Source: CAD feature listing. Evaluate the final solid. Frame: model axes, mm. Round coordinates to 2 decimals unless told otherwise and drop trailing zeros. Write each loop counter-clockwise with the first axis right and the second up, starting at its lowest first coordinate (ties: lowest second). Pieces come first, ordered by that corner, then holes. Notation, with made-up numbers: (75, 62.5) -> (97, 62.5) arc R25 ccw to (97, 86.5) -> close; hole circle Ø2 at (78, 74). An arc over 180 degrees is marked (long way). Put each result on its own line as item: value.
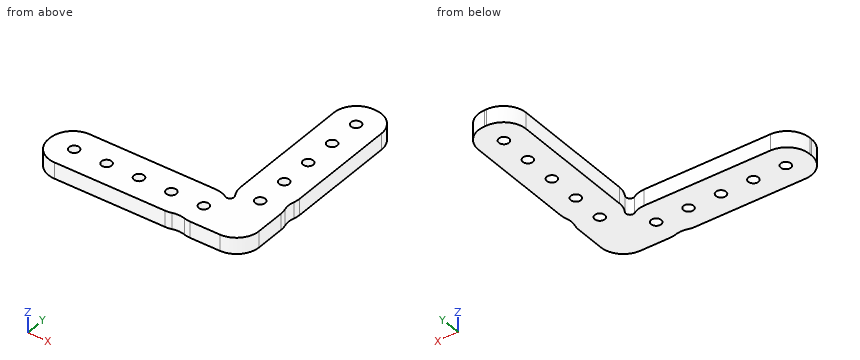
Autodesk Inventor part; units mm, degrees
ref_plane "YZ Plane" through (0, 0, 0) normal (1, 0, 0) x (0, 1, 0)
ref_plane "XZ Plane" through (0, 0, 0) normal (0, 1, 0) x (-1, 0, 0)
ref_plane "XY Plane" through (0, 0, 0) normal (0, 0, 1) x (1, 0, 0)
sketch "Sketch1" plane through (0, 0, 0) normal (0, 0, 1) x (1, 0, 0)
  line L0 (-9.3345, 9.3345) -> (-73.2155, 9.3345)
  line L1 (-73.2155, 9.3345) -> (-73.2155, -9.3345)
  line L2 (-73.2155, -9.3345) -> (9.3345, -9.3345)
  line L3 (9.3345, -9.3345) -> (9.3345, 73.2155)
  line L4 (9.3345, 73.2155) -> (-9.3345, 73.2155)
  line L5 (0, 73.2155) -> (0, 0) construction
  line L6 (0, 0) -> (-73.2155, 0) construction
  line L7 (-9.3345, 73.2155) -> (-9.3345, 9.3345)
  line L8 (-12.7, 12.7) -> (-76.581, 12.7) construction
  line L9 (-76.581, 12.7) -> (-76.581, -12.7) construction
  line L10 (-76.581, -12.7) -> (12.7, -12.7) construction
  line L11 (12.7, -12.7) -> (12.7, 76.581) construction
  line L12 (12.7, 76.581) -> (-12.7, 76.581) construction
  line L13 (-12.7, 76.581) -> (-12.7, 12.7) construction
  line L14 (9.3345, -9.3345) -> (-9.3345, 9.3345) construction
  arc A0 (-10.922, 9.3345) -> (-9.3345, 10.922) centre (-9.3345, 9.3345) ccw
  circle A1 centre (17.272, 16.0655) radius 8.636
  circle A2 centre (-16.0655, -17.272) radius 8.636
  point P0 (9.3345, 12.6631)
  point P1 (9.3345, 19.4679)
  point P2 (-19.4679, -9.3345)
  point P3 (-12.6631, -9.3345)
  dimension "d1" = 18.669
  dimension "d2" = 82.55
  dimension "d14" = 25.4
  dimension "d48" = 1.5875
  dimension "d57" = 7.9375
  dimension "d58" = 17.272
  dimension "d59" = 25.4
extrude "Plate1" add sketch "Sketch1" along normal mid plane 6.35 contours A0 L7 L4 L3 A1 L2 A2 L1 L0
sketch "Sketch3" plane through (0, 0, -3.175) normal (0, 0, -1) x (-1, 0, 0)
  line L0 (0, 0) -> (0, 73.2155) construction
  line L1 (-9.3345, 73.2155) -> (9.3345, 73.2155) construction
  line L2 (73.2155, -9.3345) -> (-9.3345, -9.3345) construction
  point P0 (0, 12.7)
  point P1 (0, 25.4)
  point P2 (0, 38.1)
  point P3 (0, 50.8)
  point P4 (0, 63.5)
  dimension "d33" = 22.0345
  dimension "d36" = 12.7
hole "Hole3" at (0, 12.7, -3.175) at (0, 25.4, -3.175) at (0, 38.1, -3.175) at (0, 50.8, -3.175) at (0, 63.5, -3.175) direction (0, 0, 1) diameter 3.9624 end through all
pattern_circular "Circular Pattern1" count 2 over 90 about axis through (0, 0, -10) along (0, 0, 1) of "Hole3"
fillet "Corner Round1" radius 8.89 11 edges at (-9.3345, 73.2155, 0) (9.3345, 73.2155, 0) (-9.3345, 10.922, 0) (9.3345, -9.3345, 0) (-73.2155, 9.3345, 0) (-73.2155, -9.3345, 0) (-10.922, 9.3345, 0) (-19.4679, -9.3345, 0) (-12.6631, -9.3345, 0) (9.3345, 19.4679, 0) (9.3345, 12.6631, 0)
equation "\"d32\" = Thickness"
equation "\"BendRadius\" = Thickness"
equation "\"BendReliefWidth\" = Thickness"
equation "\"BendReliefDepth\" = 0.5 * Thickness"
equation "\"CornerReliefSize\" = 4 * Thickness"
equation "\"MinimumRemnant\" = 2 * Thickness"
equation "\"TransitionRadius\" = BendRadius"
equation "\"JacobiRadiusSize\" = BendRadius"
equation "\"GapSize\" = Thickness"
properties part number "PLATE,BRACKET,ELEVATOR,STAGE1" material "Aluminum 7075"
Q1. Cut plane A-A on x = -25.4. Output: boundary loops of the cut face in (y, z) (1 decimal).
Ans:
outline: (-9.3, -3.2) -> (-2, -3.2) -> (-2, 3.2) -> (-9.3, 3.2) -> close; (2, -3.2) -> (9.3, -3.2) -> (9.3, 3.2) -> (2, 3.2) -> close
Q2. Material intervals for line 1 (Y direction, x = 0, z = 1.5); line 2 (X direction, y = 0, z = -0.5); line 3 (Y direction, x = -38.1, z = 0.5), sorted ascending. Write a range as [from, to].
Ans:
line 1: y = [-9.33, 10.72], [14.68, 23.42], [27.38, 36.12], [40.08, 48.82], [52.78, 61.52], [65.48, 73.22]
line 2: x = [-73.22, -65.48], [-61.52, -52.78], [-48.82, -40.08], [-36.12, -27.38], [-23.42, -14.68], [-10.72, 9.33]
line 3: y = [-9.33, -1.98], [1.98, 9.33]
Q3. Pin query (flat end, axial travel): pin 1 (1 mm diameter, centred on y = 56.5, z = 1.5, fed in from -X). Return the tip coordinate at first contact, or that it passes through.
Ans:
pin 1: stops at x = -9.33
Q4. Cut plane C-C on y = 37.5. Output: boundary loops of the cut face in (x, z) (1 decimal).
Ans:
outline: (-9.3, -3.2) -> (-1.9, -3.2) -> (-1.9, 3.2) -> (-9.3, 3.2) -> close; (1.9, -3.2) -> (9.3, -3.2) -> (9.3, 3.2) -> (1.9, 3.2) -> close
Q5. Cut plane D-D on y = 22. Output: boundary loops of the cut face in (x, z) (1 decimal).
Ans:
outline: (-9.3, -3.2) -> (9.3, -3.2) -> (9.3, 3.2) -> (-9.3, 3.2) -> close
Q6. Cut plane B-B on z = -1.5. Give the number of separate pieces and of enclosed holes in the cut face, and give its area (3 significant figures).
Ans:
separate pieces: 1
enclosed holes: 10
area: 2,510 mm^2
